For this review, take the finished solid that the model builds, in its own axes (mm). Round coordinates to 2 decimals unless told otherwise and drop trailing zeros. Answer as a JSON object with one key per item and string values.
from build123d import *

# Parameters (mm, degrees)
F0_R     = 11
F1_DEPTH = 10


# Not quite as in the source:
# - ends of sketch curves that miss each other by under 0.0002 mm in the source are joined


with BuildPart() as f1:
    # F0 (on Top) → F1 (new body)
    with BuildSketch(Plane.XY):
        with BuildLine():
            add(Edge.make_bspline(
                [(-45.9731322266, -9.229160229), (-43.4071259384, -8.4900716571), (-40.8523723257, -7.7580834253), (-38.3590158595, -7.002148962)],
                knots=[0, 0, 0, 0, 0.0911278571, 0.0911278571, 0.0911278571, 0.0911278571], degree=3))
            ThreePointArc((-45.9731322266, -9.229160229), (-51.0954988233, -29.5), (-30.9792533273, -35.1993202853))
            add(Edge.make_bspline(
                [(-30.9792533273, -35.1993202853), (-29.0552189861, -33.3450108014), (-27.1429808317, -31.496831403), (-25.2406198636, -29.713928552)],
                knots=[0, 0, 0, 0, 0.0911399969, 0.0911399969, 0.0911399969, 0.0911399969], degree=3))
            ThreePointArc((-25.2406198636, -29.713928552), (-23.6488480446, -26.0020326995), (-23.1051177665, -22))
            ThreePointArc((-23.1051177665, -22), (-27.5886656888, -11.3040084285), (-38.3590158595, -7.002148962))
        make_face()
        with Locations((-38.1051177665, -22)):
            Circle(F0_R, mode=Mode.SUBTRACT)
        with BuildLine():
            add(Edge.make_bspline(
                [(-38.3590158595, -7.002148962), (-27.1330019101, -3.5986521316), (-17.1515902552, 0.2902668448), (-12.9914200153, 7.4981996163)],
                knots=[0.0911278571, 0.0911278571, 0.0911278571, 0.0911278571, 0.5014192088, 0.5014192088, 0.5014192088, 0.5014192088], degree=3))
            ThreePointArc((-38.3590158595, -7.002148962), (-27.5886656888, -11.3040084285), (-23.1051177665, -22))
            ThreePointArc((-23.1051177665, -22), (-23.6488480446, -26.0020326995), (-25.2406198636, -29.713928552))
            add(Edge.make_bspline(
                [(-25.2406198636, -29.713928552), (-16.6860428704, -21.6965333438), (-8.3311964125, -14.9991213274), (-0.001581884, -14.9999997526)],
                knots=[0.0911399969, 0.0911399969, 0.0911399969, 0.0911399969, 0.5009802604, 0.5009802604, 0.5009802604, 0.5009802604], degree=3))
            ThreePointArc((-0.001581884, -14.9999997526), (-12.9902568617, -7.5002151081), (-12.9914200153, 7.4981996163))
        make_face()
        with BuildLine():
            add(Edge.make_bspline(
                [(-12.9914200153, 7.4981996163), (-12.9910736554, 7.4987997212), (-8.7775182768, 14.8003583601), (-10.5373469555, 25.5076949363), (-13.2795920522, 37.0248702573)],
                knots=[0.5014192088, 0.5014192088, 0.5014192088, 0.5014192088, 0.5014533681, 0.9170240175, 0.9170240175, 0.9170240175, 0.9170240175], degree=3))
            ThreePointArc((-12.9914200153, 7.4981996163), (-0.000790756, 14.9999999792), (12.9906296223, 7.4995694554))
            add(Edge.make_bspline(
                [(13.2855190223, 37.0361659764), (10.5442311657, 25.5033031012), (8.7843940058, 14.7858120219), (12.9905467554, 7.4997129635), (12.9906296223, 7.4995694554)],
                knots=[0.082935592, 0.082935592, 0.082935592, 0.082935592, 0.499552834, 0.4995610405, 0.4995610405, 0.4995610405, 0.4995610405], degree=3))
            ThreePointArc((13.2855190223, 37.0361659764), (0.0063781315, 29.000001356), (-13.2795920522, 37.0248702573))
        make_face()
        with BuildLine():
            ThreePointArc((12.9906296223, 7.4995694554), (-0.000790756, 14.9999999792), (-12.9914202607, 7.498199758))
            ThreePointArc((-12.9914202607, 7.498199758), (-12.9902568617, -7.5002151081), (-0.001581884, -14.9999999166))
            ThreePointArc((-0.001581884, -14.9999999166), (10.6060424226, -10.6071609835), (15, 0))
            ThreePointArc((15, 0), (14.4889517277, 3.8820455732), (12.9906296223, 7.4995694554))
        make_face()
        Circle(F0_R, mode=Mode.SUBTRACT)
        with BuildLine():
            ThreePointArc((15, 0), (10.6060424226, -10.6071609835), (-0.001581884, -14.9999999166))
            add(Edge.make_bspline(
                [(-0.001581884, -14.9999999166), (-0.0010545892, -14.9999998083), (8.4030291654, -15.0013139041), (16.7814390471, -21.8215724341), (25.3649320041, -29.9175543408)],
                knots=[0.5009802604, 0.5009802604, 0.5009802604, 0.5009802604, 0.5010062047, 0.9144846967, 0.9144846967, 0.9144846967, 0.9144846967], degree=3))
            ThreePointArc((25.3649320041, -29.9175543408), (25.119350955, -14.4920135645), (38.6102651526, -7.008508209))
            add(Edge.make_bspline(
                [(12.9906296082, 7.4995694472), (17.1802492182, 0.2423799612), (27.2886260541, -3.6105886019), (38.6102651526, -7.008508209)],
                knots=[0.4995610405, 0.4995610405, 0.4995610405, 0.4995610405, 0.914537264, 0.914537264, 0.914537264, 0.914537264], degree=3))
            ThreePointArc((12.9906296082, 7.4995694472), (14.4889517277, 3.8820455732), (15, 0))
        make_face()
        with BuildLine():
            add(Edge.make_bspline(
                [(-13.2795920522, 37.0248702573), (-13.8271294721, 39.3244766884), (-14.4138387907, 41.6564041587), (-15, 44)],
                knots=[0.9170240175, 0.9170240175, 0.9170240175, 0.9170240175, 1, 1, 1, 1], degree=3))
            ThreePointArc((-13.2795920522, 37.0248702573), (0.0063781315, 29.000001356), (13.2855190223, 37.0361659764))
            add(Edge.make_bspline(
                [(15, 44), (14.4158248487, 41.6601580392), (13.8312245488, 39.3320018523), (13.2855190223, 37.0361659764)],
                knots=[0, 0, 0, 0, 0.082935592, 0.082935592, 0.082935592, 0.082935592], degree=3))
            ThreePointArc((15, 44), (0, 59), (-15, 44))
        make_face()
        with Locations((0, 44)):
            Circle(F0_R, mode=Mode.SUBTRACT)
        with BuildLine():
            ThreePointArc((38.6102651526, -7.008508209), (25.119350955, -14.4920135645), (25.3649320041, -29.9175543408))
            add(Edge.make_bspline(
                [(25.3649320041, -29.9175543408), (27.1401634065, -31.5919590833), (28.9241895579, -33.3209501687), (30.7190564774, -35.055500704)],
                knots=[0.9144846967, 0.9144846967, 0.9144846967, 0.9144846967, 1, 1, 1, 1], degree=3))
            ThreePointArc((30.7190564774, -35.055500704), (45.6618723829, -34.9574480384), (53.1051177665, -22))
            ThreePointArc((53.1051177665, -22), (51.1281832536, -14.5568981387), (45.7184823908, -9.0757329377))
            add(Edge.make_bspline(
                [(38.6102651526, -7.008508209), (40.9419126032, -7.7082965101), (43.3250191135, -8.3887844569), (45.7184823908, -9.0757329377)],
                knots=[0.914537264, 0.914537264, 0.914537264, 0.914537264, 1, 1, 1, 1], degree=3))
        make_face()
        with Locations((38.1051177665, -22)):
            Circle(F0_R, mode=Mode.SUBTRACT)
    extrude(amount=F1_DEPTH)


solid = f1.part
1) Add section A-A on z = 4. State how many separate pieces and enclosed holes the cut face has, and give its area (3 significant figures).
Geometry check:
{"separate pieces": "1", "enclosed holes": "4", "area": "2,440 mm²"}
2) Insertion check: P1, Ø1, axis at x = 36.5, z = 7.5, coming from the +Y side; P2, Ø3, axis at y = 30, z = 6.5, coming from the +X side; P3, Ø3, axis at x = 36, z = 1, coming from the -Y side. Each pin has a flat end and moves straight along its axis. Give the tip position at first contact, or say it passes through.
Geometry check:
{"P1": "stops at y = -6.21", "P2": "stops at x = 12.05", "P3": "stops at y = -36.99"}
3) Mouldability with a two-part tool opening along Y and no side actions: class faces 1 (the cylindrical face through (-51.254, -29.218, 4.93)), 2 (the cylindrical face through (-46.834, -28.693, 4.93)), 3 (the cylindrical face through (-1.432, 54.906, 4.93)), 4 (the flat face through (8, -10, 10)) as +Y half, -Y half, draft (parallel to the pull), parting line (faces both ways), or undercut.
Geometry check:
{"face 1": "parting line", "face 2": "undercut", "face 3": "undercut", "face 4": "draft"}
4) For L1, parallel to Y at x = 0, z = 3.5; L2, parallel to X at y = -26, z = 6.75; L3, parallel to Y at x = 10, z = 2.5, list the stretches that pass through material, from the lowest coordinate up.
Geometry check:
{"L1": "y = -15 to -11, 11 to 33, 55 to 59", "L2": "x = -52.56 to -48.35, -27.86 to -21.16, 21.09 to 27.86, 48.35 to 52.56", "L3": "y = -17.87 to -4.58, 4.58 to 39.42, 48.58 to 55.18"}
